Work out the finished part from the listing and answer in its coordinate system (mm). A direction names the side the tool comes from. Coordinates: 2 decimals unless noted, no trailing zeros. Order: outer loops, then holes, each group sorted by start corner. A loop starts at its lowest first (then second) coordinate and runs counter-clockwise, first axis right, second up. Notation, with made-up numbers: (77.5, 58) - (93.5, 58) arc R16 cw to (93.5, 84) - close; hole circle Ø4 at (19, 48). An arc over 180 degrees is marked (long way). Answer as a JSON object with one key per item and string values. Group by question number.
1) Section B-B (x = 62) is taken. Give the vertices of the cut face in (y, z) (1 decimal).
2) A tool of negligible diameter and unlimited length cuts with its end or side. For faces 1 (the face through (88.933, 15.073, -1.541)), 2 (the face through (70, 39.931, -2)), 3 (the face through (64, 26, -2)), from which of +Z, -Z, +X, -X, +Y, -Y can it reach the whole face along a straight path? Write none if from no direction.
3) Section A-A (y = 16) is taken. Give the vertices of the cut face in (x, z) (3 decimals).
4) Section C-C (y = 6) is taken. Give the vertices of the cut face in (x, z) (1 decimal), plus the area to 3 significant figures.
5) Find the intervals of material crossed by line 1 along Y through (x, z) = (62, -0.6); line 2 along Y through (x, z) = (53.5, -1.15); line 3 along X through (y, z) = (26, -1.7), in increasing order.
6) Section D-D (x = 68) is taken. Give the vertices of the cut face in (y, z) (1 decimal).
7) Each of these flat-tipped pins is pushed along its axis until it touches: P1, Ø2.5, axis at x = 62, y = 28, coming from the +Z side; P2, Ø1.6, axis at x = 71, z = -1, coming from the -Y side; P3, Ø1.5, axis at y = 22.5, z = -2, coming from the +X side; P4, Ø5, axis at x = 82.05, y = 7.43, coming from the +Z side. Where does it stop, or does it pass through?
8) The mould has two halves that part along Y. Classify faces 4 (the face through (64, 6, -2)), 5 (the face through (99.507, 17.575, -1.541)), 6 (the face through (72, 18, 0)): released by +Y, released by -Y, zero draft, split by the parting line, or undercut.
from build123d import *

# Parameters (mm, degrees)
MODEL_R             = 3.875
MODEL_R_2           = 2.7
MODEL_R_3           = 2.125
BOSS_EXTRUDE1_DEPTH = 3.125
MODEL_3_R           = 4.125
MODEL_3_R_2         = 2.125
CUT_EXTRUDE1_DEPTH  = 2
FILLET1_R           = 6
FILLET2_R           = 6


with BuildPart() as part:
    # Model → Boss-Extrude1 (new body)
    with BuildSketch(Plane.XY):
        with BuildLine():
            Line((57.940219492, 39.930508181), (85.751165458, 39.930508181))
            Line((85.751165458, 39.930508181), (85.751165458, 34.091112415))
            ThreePointArc((85.751165458, 34.091112415), (87.9590359, 28.077103201), (93.457436342, 24.789156838))
            ThreePointArc((93.457436342, 24.789156838), (99.50819863, 17.430508181), (93.457436342, 10.071859524))
            ThreePointArc((93.457436342, 10.071859524), (87.9590359, 6.783913161), (85.751165458, 0.769903947))
            Line((85.751165458, 0.769903947), (85.751165458, -5.069491819))
            Line((85.751165458, -5.069491819), (57.940219492, -5.069491819))
            ThreePointArc((57.940219492, -5.069491819), (45.846452894, -4.78733661), (48.573590158, 6.998312478))
            ThreePointArc((48.573590158, 6.998312478), (55.686625956, 17.430508181), (48.573590158, 27.862703884))
            ThreePointArc((48.573590158, 27.862703884), (45.846452894, 39.648352972), (57.940219492, 39.930508181))
        make_face()
        with Locations((92.00819863, 17.430508181)):
            Circle(MODEL_R, mode=Mode.SUBTRACT)
        with Locations((52.008207521, -0.004787091)):
            Circle(MODEL_R_2, mode=Mode.SUBTRACT)
        with Locations((52.008207521, 34.865803453)):
            Circle(MODEL_R_2, mode=Mode.SUBTRACT)
        with Locations((82.050054867, 7.430508181)):
            Circle(MODEL_R_3, mode=Mode.SUBTRACT)
        with Locations((62.05010788, 7.430508181)):
            Circle(MODEL_R_3, mode=Mode.SUBTRACT)
        with Locations((82.050054867, 27.430508181)):
            Circle(MODEL_R_3, mode=Mode.SUBTRACT)
        with Locations((62.05010788, 27.430508181)):
            Circle(MODEL_R_3, mode=Mode.SUBTRACT)
    extrude(amount=-BOSS_EXTRUDE1_DEPTH)

    # Model_3 → Cut-Extrude1 (cut)
    with BuildSketch(Plane.XY):
        with Locations((82.050054867, 7.430508181)):
            Circle(MODEL_3_R)
        with Locations((82.050054867, 7.430508181)):
            Circle(MODEL_3_R_2, mode=Mode.SUBTRACT)
        with Locations((62.05010788, 7.430508181)):
            Circle(MODEL_3_R)
        with Locations((62.05010788, 7.430508181)):
            Circle(MODEL_3_R_2, mode=Mode.SUBTRACT)
        with Locations((62.05010788, 27.430508181)):
            Circle(MODEL_3_R)
        with Locations((62.05010788, 27.430508181)):
            Circle(MODEL_3_R_2, mode=Mode.SUBTRACT)
        with Locations((82.050054867, 27.430508181)):
            Circle(MODEL_3_R)
    extrude(amount=-CUT_EXTRUDE1_DEPTH, mode=Mode.SUBTRACT)

    # Fillet1
    fillet1_edges = [part.edges().sort_by_distance(p)[0] for p in [
        (85.751165458, -5.069491819, -1.5625),
        (85.751165458, 39.930508181, -1.5625),
    ]]
    fillet(fillet1_edges, radius=FILLET1_R)

    # Fillet2
    fillet2_edges = [part.edges().sort_by_distance(p)[0] for p in [
        (57.940219492, 39.930508181, -1.5625),
        (57.940219492, -5.069491819, -1.5625),
    ]]
    fillet(fillet2_edges, radius=FILLET2_R)


solid = part.part
Report:
{
 "1": {"outline": "(-5.1, -3.1) - (5.3, -3.1) - (5.3, -2) - (3.3, -2) - (3.3, 0) - (-5.1, 0) - close; (9.6, -3.1) - (25.3, -3.1) - (25.3, -2) - (23.3, -2) - (23.3, 0) - (11.6, 0) - (11.6, -2) - (9.6, -2) - close; (29.6, -3.1) - (39.9, -3.1) - (39.9, 0) - (31.6, 0) - (31.6, -2) - (29.6, -2) - close"},
 "2": {"face 1": "+Z, -Z", "face 2": "+Z, -Z, +X, +Y", "face 3": "+Z"},
 "3": {"outline": "(55.595, -3.125) - (88.407, -3.125) - (88.407, 0) - (55.595, 0) - close; (95.609, -3.125) - (99.371, -3.125) - (99.371, 0) - (95.609, 0) - close"},
 "4": {"outline": "(47, -3.1) - (60.5, -3.1) - (60.5, -2) - (58.2, -2) - (58.2, 0) - (47, 0) - close; (63.6, -3.1) - (80.5, -3.1) - (80.5, -2) - (78.2, -2) - (78.2, 0) - (65.9, 0) - (65.9, -2) - (63.6, -2) - close; (83.6, -3.1) - (87.4, -3.1) - (87.4, 0) - (85.9, 0) - (85.9, -2) - (83.6, -2) - close", "area": "88.1 mm²"},
 "5": {"line 1": "y = -5.07 to 3.31, 11.56 to 23.31, 31.56 to 39.93", "line 2": "y = -7.66 to -2.26, 2.25 to 10.78, 24.08 to 32.62, 37.12 to 42.52", "line 3": "x = 51.7 to 58.18, 65.92 to 78.18, 85.92 to 90.36"},
 "6": {"outline": "(-5.1, -3.1) - (39.9, -3.1) - (39.9, 0) - (-5.1, 0) - close"},
 "7": {"P1": "passes through", "P2": "stops at y = -5.07", "P3": "stops at x = 98.14", "P4": "stops at z = -2"},
 "8": {"face 4": "undercut", "face 5": "split by the parting line", "face 6": "zero draft"}
}
